Check sheet for the drawn part. Datum: minimum x, y, z corner. Units: mm. A direction names the side the tool comes from. Give positions to 0.01 mm unless a question says otherwise; leave off trailing zeros. Order: outer loops, then holes, each group sorted by start corner. A loop starts at its lowest first (then second) coordinate and runs counter-clockwise, first axis right, second up. Notation, with made-up numbers: M 28,-3 L 35,-3 A20 cw 35,35 Z; hole C 67.5,21.25 d1. An arc over 180 degrees is marked long. Put each result on its own line as item: value. Start each with the question number.
Q1. Section check B-B on y = 18.5. Record the cut outline in (x, z), then the cut area to 3 significant figures.
Q2. Material ranges on L1, parallel to X at y = 8.5, z = 5.75; L2, parallel to Y at x = 50.3, z = 7.5; L3, parallel to Z at x = 2.35, y = 13, recorded low to high.
Q3. Section check A-A on z = 7.5. Record the cut outline in (x, y), then the cut area to 4 significant figures.
Q4. Access from +Z, -Z, +X, -X, +Y, -Y to the whole of each face (thin tool, end or side, straight path). Record for the marked faces 4 and 5.
Q5. Section check D-D on x = 42. Record the cut outline in (y, z).
Q6. Go/stop test with a flat-tipped pin: pin 1 (7.5 mm diameter, centred on x = 19.5, z = 6, fed in from +Y). Record where the tip stops, or that it passes through.
Q7. Section check C-C on z = 12.5. Record the cut outline in (x, y), then the cut area to 3 significant figures.
Q8. Mould release check, pull along Y, two halves, no side actions. Record for the marked faces 1, 2 and 3: +Y half, -Y half, draft (parallel to the pull), parting line (faces both ways), or undercut.
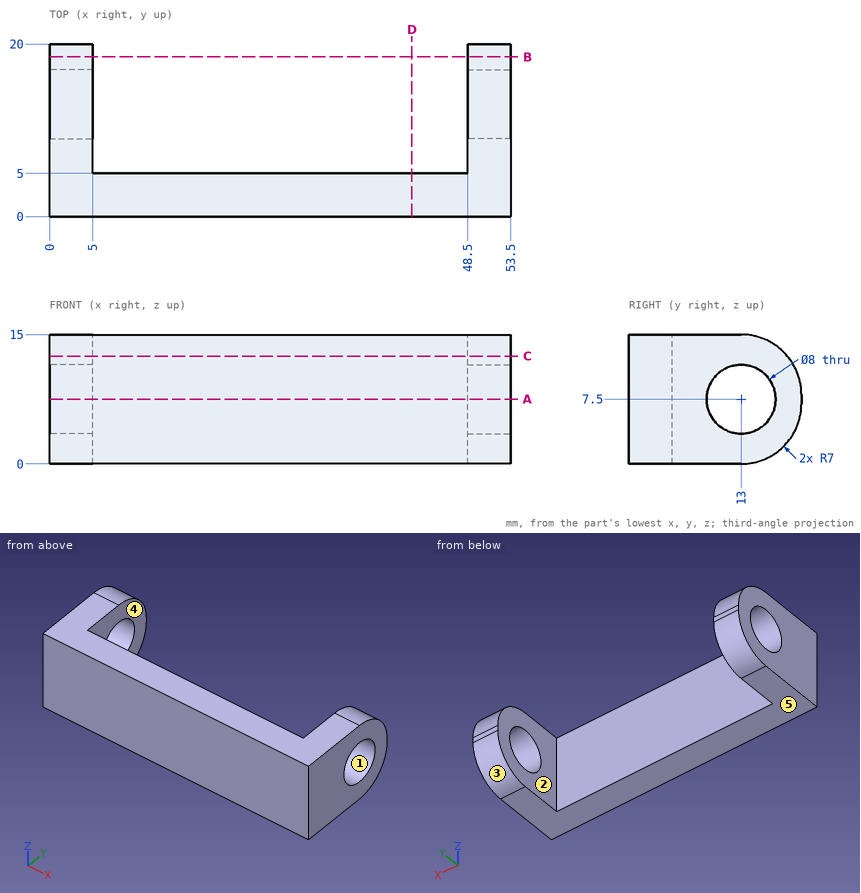
Results found:
1. outline: M 0,2.67 L 5,2.67 L 5,12.33 L 0,12.33 Z; M 48.5,2.67 L 53.5,2.67 L 53.5,12.33 L 48.5,12.33 Z
1. area: 96.6 mm^2
2. L1: x = 0 to 5, 48.5 to 53.5
2. L2: y = 0 to 9, 17 to 20
2. L3: z = 0 to 3.5, 11.5 to 15
3. outline: M 0,0 L 53.5,0 L 53.5,9 L 48.5,9 L 48.5,5 L 5,5 L 5,9 L 0,9 Z; M 0,17 L 5,17 L 5,20 L 0,20 Z; M 48.5,17 L 53.5,17 L 53.5,20 L 48.5,20 Z
3. area: 337.5 mm^2
4. face 4: +Z, -Z, +Y
4. face 5: -Z, +X, -X, +Y, -Y
5. outline: M 0,0 L 5,0 L 5,15 L 0,15 Z
6. pin 1: stops at y = 5
7. outline: M 0,0 L 53.5,0 L 53.5,18.36 L 48.5,18.36 L 48.5,5 L 5,5 L 5,18.36 L 0,18.36 Z
7. area: 401 mm^2
8. face 1: undercut
8. face 2: draft
8. face 3: +Y half
